from build123d import *

# Parameters (mm, degrees)
F1_DEPTH = 15
F2_DEPTH = 15
F3_W     = 70
F3_H     = 15
F4_DEPTH = 120
F6_DEPTH = 70


with BuildPart() as f1:
    # F0 (on Front) → F1 (new body)
    with BuildSketch(Plane.XZ):
        with BuildLine():
            Line((4, 7.5), (-4, 7.5))
            Line((-4, 7.5), (-4, -7.5))
            Line((-4, -7.5), (4, -7.5))
            ThreePointArc((4, -7.5), (-3.5, 0), (4, 7.5))
        make_face()
        with BuildLine():
            ThreePointArc((11.5, 0), (9.3033008589, 5.3033008589), (4, 7.5))
            Line((4, 7.5), (4, 4))
            ThreePointArc((4, 4), (6.8284271247, 2.8284271247), (8, 0))
            ThreePointArc((8, 0), (6.8284271247, -2.8284271247), (4, -4))
            Line((4, -4), (4, -7.5))
            ThreePointArc((4, -7.5), (9.3033008589, -5.3033008589), (11.5, 0))
        make_face()
        with BuildLine():
            Line((4, 4), (4, 7.5))
            ThreePointArc((4, 7.5), (-3.5, 0), (4, -7.5))
            Line((4, -7.5), (4, -4))
            ThreePointArc((4, -4), (0, 0), (4, 4))
        make_face()
    extrude(amount=-F1_DEPTH)

    # F2 (add): a face of the model
    f2_faces = [f1.faces().sort_by_distance(p)[0] for p in [
        (0, 0, 7.2843034539),
    ]]
    extrude(f2_faces, amount=F2_DEPTH)

    # F3 (on face) → F4 (join)
    with BuildSketch(Plane(origin=(-4, 0, 0), x_dir=(0, -1, 0), z_dir=(-1, 0, 0))):
        Rectangle(F3_W, F3_H)
    extrude(amount=F4_DEPTH)

    # F5 (on face) → F6 (join)
    with BuildSketch(Plane.XZ.offset(35)):
        Polygon((-139, -7.5), (-124, -7.5), (-124, 7.5), align=None)
    extrude(amount=-F6_DEPTH)


solid = f1.part
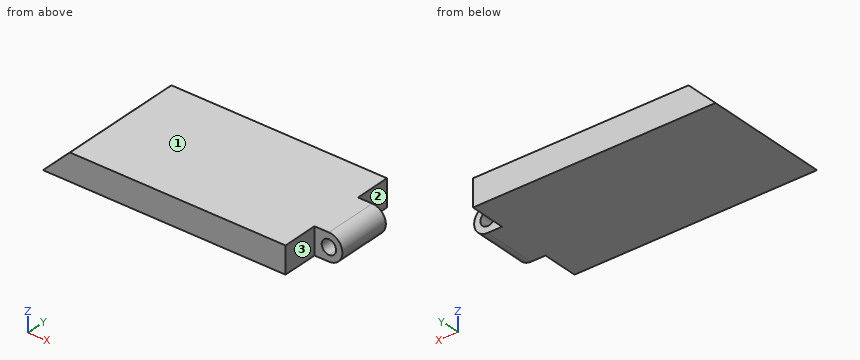
Work out the finished part from the listing and answer in its coordinate system (mm). Face numbers are marked on the shaded views. A direction names the side the tool comes from. Round coordinates to 2 decimals unless told otherwise and drop trailing zeros. Write each loop counter-clockwise with the first axis right and the second up, starting at its lowest first coordinate (ties: lowest second). Pieces come first, ordered by that corner, then holes. Notation, with made-up numbers: (13.5, -40) -> (29.5, -40) arc R23 cw to (29.5, -16) -> close; hole circle Ø6 at (-17, 75). An arc over 180 degrees is marked (long way). Write each question's results on one line, items separated by ' | '.
Item 1: Find the intervals of material crossed by line 1 along Y through (x, z) = (3.5, -7); line 2 along X through (y, z) = (-2.5, 0.75); line 3 along X through (y, z) = (-5.5, -0.75), in increasing order. Write a range as [from, to].
Result set:
line 1: [-15, 15] | line 2: [-130.75, 0.07], [7.93, 11.46] | line 3: [-132.25, 0.07], [7.93, 11.46]
Item 2: A cutting plane is placed at B-B, the plane y = -21. Determine the outline of the cut face in (x, z).
Result set:
outline: (-139, -7.5) -> (-4, -7.5) -> (-4, 7.5) -> (-124, 7.5) -> close
Item 3: Flat-ended cylindrical pins translate along their axes: P1, Ø8, axis at y = 22.5, z = 2, coming from the -X side; P2, Ø7.5, axis at y = -21, z = 1, coming from the +X side; P3, Ø4.5, axis at x = 2.5, z = -1, coming from the -Y side. Find the tip coordinate at first contact, or state that the pin passes through.
Result set:
P1: x = -133.5 | P2: x = -4 | P3: y = -15
Item 4: Which of the six approach directions +Z, -Z, +X, -X, +Y, -Y give full straight-line access (tool end or side, diameter ignored) to the marked faces 1, 2 and 3?
Result set:
face 1: +Z, +X, -X, +Y, -Y | face 2: +Z, -Z, +X, +Y | face 3: +Z, -Z, +X, -Y
Item 5: A cutting plane is placed at A-A, the plane y = -12.5. Determine the outline of the cut face in (x, z).
Result set:
outline: (-139, -7.5) -> (4, -7.5) arc R7.5 ccw to (4, 7.5) -> (-124, 7.5) -> close; hole circle Ø8 at (4, 0)
